from build123d import *

# Parameters (mm, degrees)
SKETCH1_W           = 20
SKETCH1_H           = 15
BOSS_EXTRUDE1_DEPTH = 24
CHAMFER2_SIZE       = 3
CHAMFER3_SIZE       = 3
CUT_EXTRUDE1_DEPTH  = 10


with BuildPart() as part:
    # Sketch1 → Boss-Extrude1 (new body)
    with BuildSketch(Plane.XY):
        Rectangle(SKETCH1_W, SKETCH1_H)
    extrude(amount=BOSS_EXTRUDE1_DEPTH)

    # Chamfer2
    chamfer2_edges = [part.edges().sort_by_distance(p)[0] for p in [
        (10, 0, 24),
    ]]
    chamfer(chamfer2_edges, length=CHAMFER2_SIZE)

    # Chamfer3
    chamfer3_edges = [part.edges().sort_by_distance(p)[0] for p in [
        (-10, 0, 24),
    ]]
    chamfer(chamfer3_edges, length=CHAMFER3_SIZE)

    # Sketch3 → Cut-Extrude1 (cut)
    with BuildSketch(Plane(origin=(0, 0, 0), x_dir=(-1, 0, 0), z_dir=(0, 0, -1))):
        with BuildLine():
            Line((3.122498999, 2.5), (3.122498999, -2.5))
            ThreePointArc((3.122498999, -2.5), (-4, 0), (3.122498999, 2.5))
        make_face()
    extrude(amount=-CUT_EXTRUDE1_DEPTH, mode=Mode.SUBTRACT)


solid = part.part
Geometry check sheet. Reference: the model listing, model coordinates, mm. A direction names the side the tool comes from. Round coordinates to 2 decimals unless told otherwise and drop trailing zeros. Loops run counter-clockwise (first coordinate to the right, second up) from the corner with the lowest first, then second, coordinate; pieces in that order, holes last. Notation, with made-up numbers: (-18.75, -24) -> (22.25, -24) arc R18 cw to (22.25, -11) -> close; hole circle Ø4 at (-38, 59). An arc over 180 degrees is marked (long way). Answer as a JSON object with one key per item and string values. Group by question number.
Item 1: Depth check by flat-ended pin: pin 1 Ø5.5 at (x, y) = (0, -1.5) entering from -Z. Enter the tip coordinate at first touch or a pass-through.
Item 2: Cross-section at D-D, the plane y = 5.25. Record the cut outline in (x, z), plus the area to 3 significant figures.
Item 3: Cross-section at C-C, the plane z = 6.5. Record the cut outline in (x, y), plus the area to 3 significant figures.
Item 4: Cross-section at B-B, the plane y = 0. Record the cut outline in (x, z).
Item 5: Release check for a two-part mould opening along Y. For faces 3 (the face through (4, 0, 5)), 4 (the face through (10, 0, 10)), 5 (the face through (0, 7.5, 12)), 6 (the face through (0, 0, 10)) record: pulls with the +Y half, pulls with the -Y half, needs draft (parallel to the pull), parting line crosses it, or undercut.
Item 6: Thickness scan on line 1 along Y through (x, z) = (0, 4); line 2 along X through (y, z) = (0, 5.75); line 3 along Z through (x, y) = (-1.5, 0.25). Record the ranges inside material, lowest first.
Item 7: Cross-section at A-A, the plane x = 0. Record the cut outline in (y, z).
Item 8: Set-up check for faces 1 (the face through (-3.122, 0, 5)), 2 (the face through (-2.4, 3.4, 0)): record each of +Z, -Z, +X, -X, +Y, -Y from which the full face is reachable in a straight line by a thin tool's end or side.
Determined:
{
 "1": {"pin 1": "stops at z = 0"},
 "2": {"outline": "(-10, 0) -> (10, 0) -> (10, 21) -> (7, 24) -> (-7, 24) -> (-10, 21) -> close", "area": "471 mm²"},
 "3": {"outline": "(-10, -7.5) -> (10, -7.5) -> (10, 7.5) -> (-10, 7.5) -> close; hole (-3.12, -2.5) arc R4 ccw (long way) to (-3.12, 2.5) -> close", "area": "253 mm²"},
 "4": {"outline": "(-10, 0) -> (-3.12, 0) -> (-3.12, 10) -> (4, 10) -> (4, 0) -> (10, 0) -> (10, 21) -> (7, 24) -> (-7, 24) -> (-10, 21) -> close"},
 "5": {"face 3": "undercut", "face 4": "needs draft", "face 5": "pulls with the +Y half", "face 6": "undercut"},
 "6": {"line 1": "y = -7.5 to -4, 4 to 7.5", "line 2": "x = -10 to -3.12, 4 to 10", "line 3": "z = 10 to 24"},
 "7": {"outline": "(-7.5, 0) -> (-4, 0) -> (-4, 10) -> (4, 10) -> (4, 0) -> (7.5, 0) -> (7.5, 24) -> (-7.5, 24) -> close"},
 "8": {"face 1": "-Z", "face 2": "-Z, +X, -X, +Y, -Y"}
}
